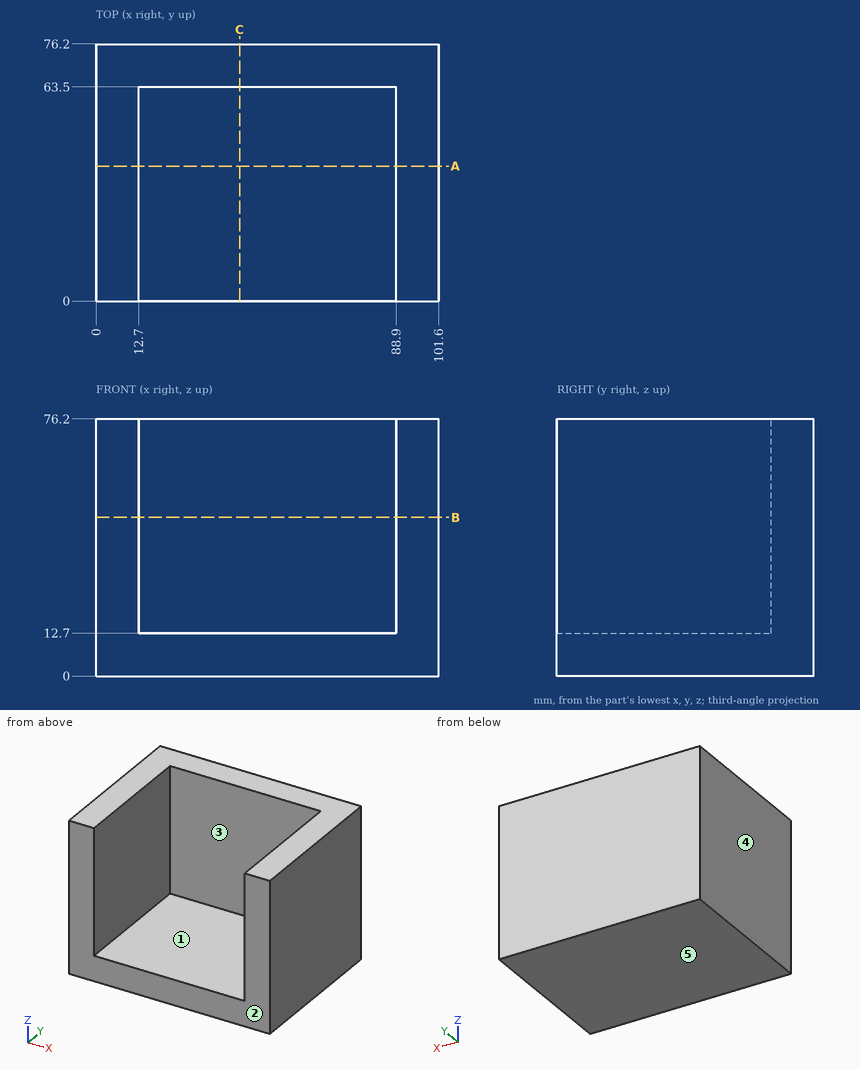
Study the drawing (mm; zero at the part's minimum x, y, z) and answer. A direction names the side the tool comes from. Give positions to 0.01 mm unless a question says otherwise; leave off trailing zeros. Loops run counter-clockwise (first coordinate to the right, second up) from the corner with the lowest first, then second, coordinate; pieces in that order, holes last. Notation, with made-up numbers: M 61.5,66.25 L 74.5,66.25 A19 cw 74.5,92.25 Z; hole C 80,69.25 d10. An arc over 180 degrees is marked long. One line per item, written item: value.
1. For a pull along X with two mould halves and no side action, classify the marked faces 3, 4 and 5 as pulls with the +X half, pulls with the -X half, needs draft (parallel to the pull), parting line crosses it, or undercut.
Found:
face 3: undercut
face 4: pulls with the -X half
face 5: needs draft
2. Section C-C on x = 42.5 is taken. Determine the outline of the cut face in (y, z).
Found:
outline: M 0,0 L 76.2,0 L 76.2,76.2 L 63.5,76.2 L 63.5,12.7 L 0,12.7 Z
3. Find the intervals of material crossed by probe 1 along X at (y, z) = (24.5, 29); probe 2 along Z at (x, y) = (54.5, 52); probe 3 along Y at (x, z) = (64, 58), in increasing order.
Found:
probe 1: 0 to 12.7, 88.9 to 101.6
probe 2: 0 to 12.7
probe 3: 63.5 to 76.2
4. For the marked faces 1 and 2, determine the directions among +Z, -Z, +X, -X, +Y, -Y from which every point of the face is accessible in a straight line to the end or side of a thin tool.
Found:
face 1: +Z, -Y
face 2: +Z, -Z, +X, -X, -Y
5. Section B-B on z = 47 is taken. Determine the outline of the cut face in (x, y), plus the area to 3 significant figures.
Found:
outline: M 0,0 L 12.7,0 L 12.7,63.5 L 88.9,63.5 L 88.9,0 L 101.6,0 L 101.6,76.2 L 0,76.2 Z
area: 2,900 mm^2
6. This flat-tipped pin is pushed along its axis until it touches: P1, Ø10, axis at x = 60.5, z = 56, coming from the -Y side. Where does it stop, or does it pass through?
Found:
P1: y = 63.5
7. Section A-A on y = 40 is taken. Determine the outline of the cut face in (x, z).
Found:
outline: M 0,0 L 101.6,0 L 101.6,76.2 L 88.9,76.2 L 88.9,12.7 L 12.7,12.7 L 12.7,76.2 L 0,76.2 Z
